Geometry: see drawing. Coordinates: mm, zero at the bounding-box minimum. Give positions to 0.01 mm unless a question says otherwise; leave off trailing zeros. Loops run counter-clockwise (first coordinate to the right, second up) from the corner with the lowest first, then second, coordinate; pieces in that order, holes last. Notation, with made-up numbers: (-15, -5.5) -> (4, -5.5) arc R15 ccw to (4, 22.5) -> close; hole circle Ø8 at (72, -39). An arc over 180 degrees is marked (long way). Return JSON: item names as keys, results as strings. Group by question number.
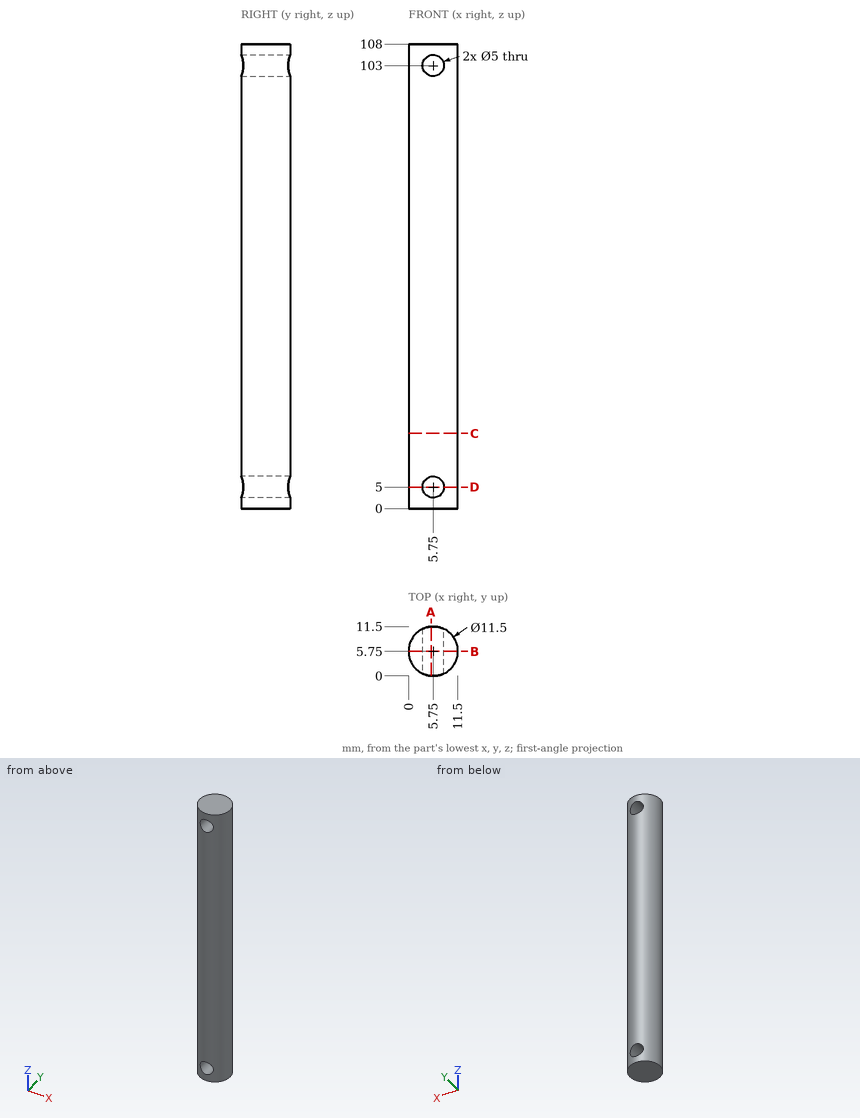
1) Cut plane B-B on y = 5.75. Return loops of the section in (x, z), then the cut area to 3 significant figures.
2) Cut plane A-A on x = 5.25. Return loops of the section in (y, z).
3) Material intervals for line 1 (Z direction, x = 5.75, y = 4.5); line 2 (Z direction, x = 5.25, y = 1.75); line 3 (X direction, y = 5.25, z = 29), sorted ascending.
4) Contact query for flat-ended pins moving along their axis: P1, Ø3, axis at y = 9, z = 40.5, coming from the -X side; P2, Ø4, axis at x = 5.75, z = 5, coming from the -Y side; P3, Ø5, axis at x = 9, z = 48, coming from the -Y side; P4, Ø1.5, axis at y = 3, z = 87, coming from the -X side. Output: stop coordinate, or through.
5) Cut plane C-C on z = 17.5. Return loops of the section in (x, y).
6) Cut plane D-D on z = 5. Return loops of the section in (x, y).
Calculated:
{
 "1": {"outline": "(0, 0) -> (11.5, 0) -> (11.5, 108) -> (0, 108) -> close; hole circle Ø5 at (5.75, 5); hole circle Ø5 at (5.75, 103)", "area": "1,200 mm2"},
 "2": {"outline": "(0.02, 0) -> (11.48, 0) -> (11.48, 2.55) -> (0.02, 2.55) -> close; (0.02, 7.45) -> (11.48, 7.45) -> (11.48, 100.55) -> (0.02, 100.55) -> close; (0.02, 105.45) -> (11.48, 105.45) -> (11.48, 108) -> (0.02, 108) -> close"},
 "3": {"line 1": "0 to 2.5, 7.5 to 100.5, 105.5 to 108", "line 2": "0 to 2.55, 7.45 to 100.55, 105.45 to 108", "line 3": "0.02 to 11.48"},
 "4": {"P1": "x = 0.27", "P2": "through", "P3": "y = 0.05", "P4": "x = 0.36"},
 "5": {"outline": "circle Ø11.5 at (5.75, 5.75)"},
 "6": {"outline": "(3.25, 0.57) -> (3.25, 10.93) arc R5.75 ccw to start; (8.25, 0.57) arc R5.75 ccw to (8.25, 10.93) -> close"}
}
